Geometry check sheet. Reference: the model listing, model coordinates, mm. A direction names the side the tool comes from. Give positions to 0.01 mm unless a question says otherwise; leave off trailing zeros. Order: outer loops, then holes, each group sorted by start corner. A loop starts at its lowest first (then second) coordinate and runs counter-clockwise, first axis right, second up.
from build123d import *

# Parameters (mm, degrees)
BOSS_EXTRUDE1_DEPTH = 6.35
CUT_EXTRUDE1_REACH  = 116.652
SKETCH2_R           = 2.4892
CUT_EXTRUDE3_REACH  = 116.652
SKETCH4_R           = 1.397
SKETCH4_R_2         = 4.7625
FILLET4_R           = 12.7
FILLET5_R           = 19.05


with BuildPart() as part:
    # Sketch1 → Boss-Extrude1 (new body)
    with BuildSketch(Plane.XY):
        Polygon((0, 0), (12.7, 0), (12.7, 50.8), (50.8, 50.8), (50.8, 0), (63.5, 0), (63.5, 63.5), (31.75, 95.25), (6.35, 95.25), (0, 82.55), align=None)
    extrude(amount=BOSS_EXTRUDE1_DEPTH)

    # Sketch2 → Cut-Extrude1 (cut, up to next)
    with BuildSketch(Plane.XY.offset(6.35), mode=Mode.PRIVATE) as cut_extrude1_sk1:
        with Locations((6.35, 12.7)):
            Circle(SKETCH2_R)
    cut_extrude1_tool1 = extrude(cut_extrude1_sk1.sketch, amount=-CUT_EXTRUDE1_REACH, mode=Mode.PRIVATE) & part.part
    # Sketch2 → Cut-Extrude1 (cut, up to next)
    with BuildSketch(Plane.XY.offset(6.35), mode=Mode.PRIVATE) as cut_extrude1_sk2:
        with Locations((6.35, 31.75)):
            Circle(SKETCH2_R)
    cut_extrude1_tool2 = extrude(cut_extrude1_sk2.sketch, amount=-CUT_EXTRUDE1_REACH, mode=Mode.PRIVATE) & part.part
    # Sketch2 → Cut-Extrude1 (cut, up to next)
    with BuildSketch(Plane.XY.offset(6.35), mode=Mode.PRIVATE) as cut_extrude1_sk3:
        with Locations((57.15, 12.7)):
            Circle(SKETCH2_R)
    cut_extrude1_tool3 = extrude(cut_extrude1_sk3.sketch, amount=-CUT_EXTRUDE1_REACH, mode=Mode.PRIVATE) & part.part
    # Sketch2 → Cut-Extrude1 (cut, up to next)
    with BuildSketch(Plane.XY.offset(6.35), mode=Mode.PRIVATE) as cut_extrude1_sk4:
        with Locations((57.15, 31.75)):
            Circle(SKETCH2_R)
    cut_extrude1_tool4 = extrude(cut_extrude1_sk4.sketch, amount=-CUT_EXTRUDE1_REACH, mode=Mode.PRIVATE) & part.part
    add(cut_extrude1_tool1.solids().sort_by_distance((6.35, 12.7, 6.35))[0], mode=Mode.SUBTRACT)
    add(cut_extrude1_tool2.solids().sort_by_distance((6.35, 31.75, 6.35))[0], mode=Mode.SUBTRACT)
    add(cut_extrude1_tool3.solids().sort_by_distance((57.15, 12.7, 6.35))[0], mode=Mode.SUBTRACT)
    add(cut_extrude1_tool4.solids().sort_by_distance((57.15, 31.75, 6.35))[0], mode=Mode.SUBTRACT)

    # Sketch4 → Cut-Extrude3 (cut, up to next)
    with BuildSketch(Plane.XY.offset(6.35), mode=Mode.PRIVATE) as cut_extrude3_sk1:
        with Locations((12.7, 52.3875)):
            Circle(SKETCH4_R)
    cut_extrude3_tool1 = extrude(cut_extrude3_sk1.sketch, amount=-CUT_EXTRUDE3_REACH, mode=Mode.PRIVATE) & part.part
    # Sketch4 → Cut-Extrude3 (cut, up to next)
    with BuildSketch(Plane.XY.offset(6.35), mode=Mode.PRIVATE) as cut_extrude3_sk2:
        with Locations((12.7, 87.3125)):
            Circle(SKETCH4_R)
    cut_extrude3_tool2 = extrude(cut_extrude3_sk2.sketch, amount=-CUT_EXTRUDE3_REACH, mode=Mode.PRIVATE) & part.part
    # Sketch4 → Cut-Extrude3 (cut, up to next)
    with BuildSketch(Plane.XY.offset(6.35), mode=Mode.PRIVATE) as cut_extrude3_sk3:
        with Locations((38.1, 69.85)):
            Circle(SKETCH4_R_2)
    cut_extrude3_tool3 = extrude(cut_extrude3_sk3.sketch, amount=-CUT_EXTRUDE3_REACH, mode=Mode.PRIVATE) & part.part
    add(cut_extrude3_tool1.solids().sort_by_distance((12.7, 52.3875, 6.35))[0], mode=Mode.SUBTRACT)
    add(cut_extrude3_tool2.solids().sort_by_distance((12.7, 87.3125, 6.35))[0], mode=Mode.SUBTRACT)
    add(cut_extrude3_tool3.solids().sort_by_distance((38.1, 69.85, 6.35))[0], mode=Mode.SUBTRACT)

    # Fillet4
    fillet4_edges = [part.edges().sort_by_distance(p)[0] for p in [
        (50.8, 50.8, 3.175),
        (12.7, 50.8, 3.175),
    ]]
    fillet(fillet4_edges, radius=FILLET4_R)

    # Fillet5
    # the kernel refuses this fillet: 19.05 mm, written as the material it takes off along each edge
    with BuildSketch(Plane(origin=(0, 82.55, -11.242737428), x_dir=(0, -1, 0), z_dir=(0, 0, 1))) as fillet5_piece_1:
        with BuildLine():
            CenterArc((FILLET5_R * 0.2360679775, FILLET5_R), FILLET5_R, 243.434948823, 26.565051177)
            Line((-FILLET5_R * 0.211145618, FILLET5_R * 0.105572809), (0, 0))
            Line((0, 0), (FILLET5_R * 0.2360679775, 0))
        make_face()
    extrude(amount=28.835474857, mode=Mode.SUBTRACT)
    with BuildSketch(Plane(origin=(6.35, 95.25, -29.433868714), x_dir=(-0.4472135954999575, -0.8944271909999162, 0), z_dir=(0, 0, 1))) as fillet5_piece_2:
        with BuildLine():
            CenterArc((FILLET5_R * 0.61803398875, FILLET5_R), FILLET5_R, 206.565051177, 63.434948823)
            Line((-FILLET5_R * 0.27639320225, FILLET5_R * 0.5527864045), (0, 0))
            Line((0, 0), (FILLET5_R * 0.61803398875, 0))
        make_face()
    extrude(amount=65.217737428, mode=Mode.SUBTRACT)
    with BuildSketch(Plane(origin=(31.75, 95.25, -19.726920908), x_dir=(-1, 0, 0), z_dir=(0, 0, 1)), Plane(origin=(63.5, 63.5, -19.726920908), x_dir=(-0.7071067811865476, 0.7071067811865476, 0), z_dir=(0, 0, 1))) as fillet5_piece_3:
        with BuildLine():
            CenterArc((FILLET5_R * 0.414213562373, FILLET5_R), FILLET5_R, 225, 45)
            Line((-FILLET5_R * 0.292893218813, FILLET5_R * 0.292893218813), (0, 0))
            Line((0, 0), (FILLET5_R * 0.414213562373, 0))
        make_face()
    extrude(amount=45.803841816, mode=Mode.SUBTRACT)


solid = part.part
Item 1: Draft check along X on faces 3 (the flat face through (0, 40, 3)), 4 (the flat face through (31, 59, 0)), 5 (the cylindrical face through (8.724, 32.498, 3.219)). Enter one of: released by +X, released by -X, zero draft, split by the parting line, or undercut.
Reported:
face 3: released by -X
face 4: zero draft
face 5: undercut
Item 2: Gauge pin test, flat ends, axial feed: pin 1 (15 mm diameter, centred on x = 38.1, y = 69.85, fed in from +Z); pin 2 (1.7 mm diameter, centred on x = 12.7, y = 52.39, fed in from +Z). Record the tip position at first contact, or that the pin passes through.
Reported:
pin 1: stops at z = 6.35
pin 2: passes through
Item 3: Scan lines: L1, parallel to X at y = 31.5, z = 3.25; L2, parallel to Y at x = 57, z = 5.5; L3, parallel to Y at x = 57.15, z = 3.75. Record each from-to range of solid material in increasing order.
Reported:
L1: x = 0 to 3.87, 8.83 to 12.7, 50.8 to 54.67, 59.63 to 63.5
L2: y = 0 to 10.22, 15.18 to 29.27, 34.23 to 70
L3: y = 0 to 10.21, 15.19 to 29.26, 34.24 to 69.85
Item 4: Sectioned sample at B-B (x = 6.35). Enter the section's corners in (y, z), and give its area (3 significant figures).
Reported:
outline: (0, 0) - (10.21, 0) - (10.21, 6.35) - (0, 6.35) - close; (15.19, 0) - (29.26, 0) - (29.26, 6.35) - (15.19, 6.35) - close; (34.24, 0) - (91.18, 0) - (91.18, 6.35) - (34.24, 6.35) - close
area: 516 mm2
Item 5: Sectioned sample at D-D (y = 76). Enter the section's corners in (x, z).
Reported:
outline: (0, 0) - (51, 0) - (51, 6.35) - (0, 6.35) - close
Item 6: Sectioned sample at C-C (z = 1.25). Give the number of separate pieces and of enclosed holes in the cut face, and give its area (3 significant figures).
Reported:
separate pieces: 1
enclosed holes: 7
area: 3,440 mm2
Item 7: Sectioned sample at A-A (y = 31.75). Enter the section's corners in (x, z).
Reported:
outline: (0, 0) - (3.86, 0) - (3.86, 6.35) - (0, 6.35) - close; (8.84, 0) - (12.7, 0) - (12.7, 6.35) - (8.84, 6.35) - close; (50.8, 0) - (54.66, 0) - (54.66, 6.35) - (50.8, 6.35) - close; (59.64, 0) - (63.5, 0) - (63.5, 6.35) - (59.64, 6.35) - close
Item 8: Set-up check for faces 1 (the cylindrical face through (31.25, 93.76, 3.13)), 2 (the cylindrical face through (16.32, 46.98, 3.22)): record each of +Z, -Z, +X, -X, +Y, -Y from which the full face is reachable in a straight line by a thin tool's end or side.
Reported:
face 1: +Z, -Z, +X, +Y
face 2: +Z, -Z, -Y
